from build123d import *

# Parameters (mm, degrees)
BOSS_EXTRUDE1_DEPTH = 38.1
SKETCH2_R           = 11.049
CUT_EXTRUDE1_DEPTH  = 6.35
SKETCH2_4_R         = 3.556
CUT_EXTRUDE2_DEPTH  = 6.35


with BuildPart() as part:
    # Sketch1 → Boss-Extrude1 (new body)
    with BuildSketch(Plane.XY):
        Polygon((0, 76.2), (0, 0), (6.35, 0), (6.35, 69.85), (6.35, 76.2), align=None)
        Polygon((88.097991824, 76.2), (6.35, 76.2), (6.35, 69.85), (94.447991824, 69.85), (94.447991824, 101.6), (88.097991824, 101.6), align=None)
    extrude(amount=BOSS_EXTRUDE1_DEPTH)

    # Sketch2 → Cut-Extrude1 (cut)
    with BuildSketch(Plane.ZY):
        with Locations((19.05, 20.32)):
            Circle(SKETCH2_R)
    extrude(amount=-CUT_EXTRUDE1_DEPTH, mode=Mode.SUBTRACT)

    # Sketch2_4 → Cut-Extrude2 (cut)
    with BuildSketch(Plane.ZY):
        with Locations((19.05, 42.672)):
            Circle(SKETCH2_4_R)
    extrude(amount=-CUT_EXTRUDE2_DEPTH, mode=Mode.SUBTRACT)


solid = part.part
Model file for the job. Use its own axes, mm. A direction names the side the tool comes from. Round coordinates to 2 decimals unless told otherwise and drop trailing zeros. Loops run counter-clockwise (first coordinate to the right, second up) from the corner with the lowest first, then second, coordinate; pieces in that order, holes last.
1. Wall check: probe 1 along Y at (x, z) = (5, 19); probe 2 along Z at (x, y) = (3, 20); probe 3 along Y at (x, z) = (86, 18). Give the ranges that are in metal, low to high.
Check values:
probe 1: y = 0 to 9.27, 31.37 to 39.12, 46.23 to 76.2
probe 2: z = 0 to 8.01, 30.09 to 38.1
probe 3: y = 69.85 to 76.2
2. Band-saw the part on B-B, the plane y = 20.32. List the corners of the cut face in (x, z).
Check values:
outline: (0, 0) - (6.35, 0) - (6.35, 8) - (0, 8) - close; (0, 30.1) - (6.35, 30.1) - (6.35, 38.1) - (0, 38.1) - close
3. Band-saw the part on D-D, the plane x = 37.5. List the corners of the cut face in (y, z).
Check values:
outline: (69.85, 0) - (76.2, 0) - (76.2, 38.1) - (69.85, 38.1) - close
4. Mould opens along Z. For faces 1 (the cylindrical face through (3.13, 13.6, 10.28)), 2 (the flat face through (37, 70, 0)), 3 (the cylindrical face through (3.13, 39.2, 18.28)), 4 (the flat face through (50, 69.85, 19)) say: +Z half, -Z half, draft (parallel to the pull), parting line (faces both ways), or undercut.
Check values:
face 1: undercut
face 2: -Z half
face 3: undercut
face 4: draft
5. Drop flat-ended pins along their axis: P1, Ø9, axis at y = 42.672, z = 19.05, coming from the +X side; P2, Ø10, axis at x = 46, z = 5.5, coming from the +Y side; P3, Ø3, axis at x = 48, z = 17, coming from the -Y side; P4, Ø13.5, axis at y = 20.32, z = 19.05, coming from the +X side. Give the stop position or say it passes through.
Check values:
P1: stops at x = 6.35
P2: stops at y = 76.2
P3: stops at y = 69.85
P4: passes through
6. Band-saw the part on C-C, the plane z = 32.5. List the corners of the cut face in (x, y).
Check values:
outline: (0, 0) - (6.35, 0) - (6.35, 69.85) - (94.45, 69.85) - (94.45, 101.6) - (88.1, 101.6) - (88.1, 76.2) - (0, 76.2) - close
7. Tool access for faces 5 (the flat face through (88.098, 89, 19)), 6 (the flat face through (3, 0, 19)), 7 (the flat face through (6.35, 34, 19)): list every direction of +Z, -Z, +X, -X, +Y, -Y with a clear straight run to the whole face (end or side of a thin tool).
Check values:
face 5: +Z, -Z, -X, +Y
face 6: +Z, -Z, +X, -X, -Y
face 7: +Z, -Z, +X, -Y
8. Band-saw the part on A-A, the plane z = 19.05. List the corners of the cut face in (x, y).
Check values:
outline: (0, 0) - (6.35, 0) - (6.35, 9.27) - (0, 9.27) - close; (0, 31.37) - (6.35, 31.37) - (6.35, 39.12) - (0, 39.12) - close; (0, 46.23) - (6.35, 46.23) - (6.35, 69.85) - (94.45, 69.85) - (94.45, 101.6) - (88.1, 101.6) - (88.1, 76.2) - (0, 76.2) - close
